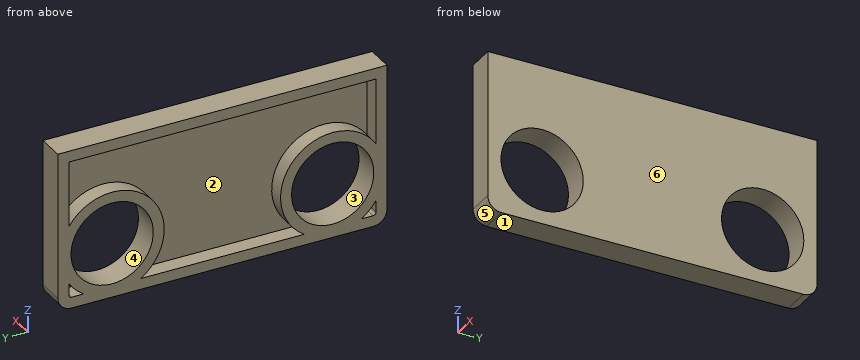
from build123d import *

# Parameters (mm, degrees)
F0_W     = 13.5
F0_H     = 6.75
F1_DEPTH = 20
F2_W     = 8
F2_H     = 26.4694701647
F3_DEPTH = 12
F4_R     = 0.49999
F7_R     = 7.5
F8_DEPTH = 5
F9_T     = -2


# Not quite as in the source:
# - a fillet or chamfer is up to 0.001 mm smaller than in the source, because OpenCascade refuses the exact size
# - a feature of the source that left no trace in its solid (it failed there, or was rolled back) is left out


with BuildPart() as f1:
    # F0 (on Right) → F1 (new body)
    with BuildSketch(Plane.YZ):
        with BuildLine():
            Line((21.2005410668, -21.2570374378), (21.2005410668, 3.4429625622))
            Line((21.2005410668, 3.4429625622), (24.7505410668, 3.4429625622))
            Line((24.7505410668, 3.4429625622), (24.7505410668, -5.3425713437))
            Line((24.7505410668, -5.3425713437), (24.7505410668, -14.0570374378))
            ThreePointArc((24.7505410668, -14.0570374378), (25.4827741138, -15.8248043907), (27.2505410668, -16.5570374378))
            Line((27.2505410668, -16.5570374378), (31.4505410668, -16.5570374378))
            ThreePointArc((31.4505410668, -16.5570374378), (33.2183080197, -15.8248043907), (33.9505410668, -14.0570374378))
            Line((33.9505410668, -14.0570374378), (33.9505410668, -5.3425713437))
            Line((33.9505410668, -5.3425713437), (33.9505410668, 6.3718947504))
            ThreePointArc((33.9505410668, 6.3718947504), (34.4092996144, 7.8152704233), (35.6172077334, 8.7289173543))
            ThreePointArc((35.6172077334, 8.7289173543), (37.4860749727, 16.9784964681), (29.2364958588, 15.1096292289))
            ThreePointArc((29.2364958588, 15.1096292289), (28.3228489279, 13.9017211099), (26.8794732549, 13.4429625622))
            Line((26.8794732549, 13.4429625622), (15.2005410668, 13.4429625622))
            Line((15.2005410668, 13.4429625622), (-1.2994589332, 13.4429625622))
            ThreePointArc((-1.2994589332, 13.4429625622), (-3.0672258862, 12.7107295152), (-3.7994589332, 10.9429625622))
            Line((-3.7994589332, 10.9429625622), (-3.7994589332, 5.9429625622))
            ThreePointArc((-3.7994589332, 5.9429625622), (-3.0672258862, 4.1751956093), (-1.2994589332, 3.4429625622))
            Line((-1.2994589332, 3.4429625622), (5.1650071608, 3.4429625622))
            ThreePointArc((5.1650071608, 3.4429625622), (6.1217157417, 3.2526613935), (6.9327741138, 2.7107295152))
            Line((6.9327741138, 2.7107295152), (14.4934342856, -4.8499306566))
            Line((14.4934342856, -4.8499306566), (15.4683080197, -5.8248043907))
            ThreePointArc((15.4683080197, -5.8248043907), (16.010239898, -6.6358627628), (16.2005410668, -7.5925713437))
            Line((16.2005410668, -7.5925713437), (16.2005410668, -21.2570374378))
            ThreePointArc((16.2005410668, -21.2570374378), (16.4934342856, -21.964144219), (17.2005410668, -22.2570374378))
            Line((17.2005410668, -22.2570374378), (20.2005410668, -22.2570374378))
            ThreePointArc((20.2005410668, -22.2570374378), (20.9076478479, -21.964144219), (21.2005410668, -21.2570374378))
        make_face()
        with Locations((5.7005410668, 7.8179625622)):
            Rectangle(F0_W, F0_H, mode=Mode.SUBTRACT)
    extrude(amount=F1_DEPTH)

    # F2 (on face) → F3 (cut)
    with BuildSketch(Plane.YZ.offset(20)):
        with Locations((5.7005410668, 11.1929625622)):
            Rectangle(F2_W, F2_H)
    extrude(amount=-F3_DEPTH, mode=Mode.SUBTRACT)

    # F4 (radius 0.5 in the source; OpenCascade refuses exactly that, so slightly less here)
    f4_edges = [f1.edges().sort_by_distance(p)[0] for p in [
        (14, 1.700541, 11.192963),
        (14, 1.700541, 13.442963),
        (14, 1.700541, 4.442963),
        (14, 1.700541, 3.442963),
        (10, -1.049459, 4.442963),
        (10, -1.049459, 11.192963),
        (10, 12.450541, 11.192963),
        (10, 12.450541, 4.442963),
        (14, 9.700541, 11.192963),
        (14, 9.700541, 13.442963),
        (14, 9.700541, 4.442963),
    ]]
    fillet(f4_edges, radius=F4_R)


with BuildPart() as f8:
    # F7 (on Right) → F8 (new body)
    with BuildSketch(Plane.YZ):
        with BuildLine():
            Line((-17.6103499532, 45.065652512), (-22.6103499532, 45.065652512))
            Line((-22.6103499532, 45.065652512), (-72.6103499532, 45.065652512))
            Line((-72.6103499532, 45.065652512), (-77.6103499532, 45.065652512))
            Line((-77.6103499532, 45.065652512), (-77.6103499532, 27.565652512))
            ThreePointArc((-77.6103499532, 27.565652512), (-76.8781169061, 25.7978855591), (-75.1103499532, 25.065652512))
            Line((-75.1103499532, 25.065652512), (-20.1103499532, 25.065652512))
            ThreePointArc((-20.1103499532, 25.065652512), (-18.3425830002, 25.7978855591), (-17.6103499532, 27.565652512))
            Line((-17.6103499532, 27.565652512), (-17.6103499532, 45.065652512))
        make_face()
        with Locations((-67.7103499532, 35.015652512)):
            Circle(F7_R, mode=Mode.SUBTRACT)
        with Locations((-27.5103499532, 35.015652512)):
            Circle(F7_R, mode=Mode.SUBTRACT)
        Polygon((-72.6103499532, 45.065652512), (-22.6103499532, 45.065652512), (-17.6103499532, 45.065652512), (-17.6103499532, 54.265652512), (-77.6103499532, 54.265652512), (-77.6103499532, 45.065652512), align=None)
    extrude(amount=F8_DEPTH)

    # F9
    f9_openings = [f8.faces().sort_by_distance(p)[0] for p in [
        (0, -47.61035, 40.869984),
    ]]
    offset(amount=F9_T, openings=f9_openings)


solid = f8.part
Read the model definition and answer for the solid it produces. Units are mm, in the model's axes. Face numbers are marked on the shaded views. A direction names the side the tool comes from. Round coordinates to 2 decimals unless told otherwise and drop trailing zeros. Order: outer loops, then holes, each group sorted by start corner. A loop starts at its lowest first (then second) coordinate and runs counter-clockwise, first axis right, second up.
1) Flat-ended cylindrical pins translate along their axes: pin 1 (7.5 mm diameter, centred on y = -55.5, z = 41.5, fed in from -X); pin 2 (9 mm diameter, centred on y = -27.51, z = 35.02, fed in from -X). Find the tip coordinate at first contact, or state that the pin passes through.
2) Straight lines are drawn through the part: L1, parallel to Z at x = 2.1, y = -68; L2, parallel to Z at x = 0.3, y = -34; L3, parallel to Z at x = 1.5, y = -62. For each, find the intervals that lie inside material, in ascending order.
3) For the marked faces 1 and 2, determine the directions among +Z, -Z, +X, -X, +Y, -Y from which every point of the face is accessible in a straight line to the end or side of a thin tool.
4) The part is cut by section A-A on z = 33. Write down the section's boundary in (x, y), plus the area to 3 significant figures.
5) The part is cut by section D-D on y = -49.5. Write down the section's boundary in (x, z).
6) The part is cut by section B-B on y = -74. Write down the section's boundary in (x, z), plus the area to 3 significant figures.
7) The mould has two halves that part along Y. Classify the marked faces 3, 4, 5 and 6: released by +Y, released by -Y, zero draft, split by the parting line, or undercut.
8) The part is cut by section C-C on x = 0.6. Write down the section's boundary in (y, z), plus the area to 3 significant figures.
Resolved:
1. pin 1: stops at x = 3
1. pin 2: passes through
2. L1: z = 25.07 to 27.52, 42.51 to 44.51, 52.27 to 54.27
2. L2: z = 25.07 to 27.07, 28.08 to 31.26, 38.78 to 41.95, 52.27 to 54.27
2. L3: z = 25.07 to 27.07, 27.42 to 30.15, 39.88 to 42.61, 52.27 to 54.27
3. face 1: -Z, +X, -X, +Y, -Y
3. face 2: -X
4. outline: (0, -77.61) - (5, -77.61) - (5, -74.93) - (0, -74.93) - close; (0, -60.49) - (5, -60.49) - (5, -34.73) - (0, -34.73) - (0, -36.79) - (3, -36.79) - (3, -58.43) - (0, -58.43) - close; (0, -20.29) - (5, -20.29) - (5, -17.61) - (0, -17.61) - close
4. area: 90.6 mm2
5. outline: (0, 25.07) - (5, 25.07) - (5, 54.27) - (0, 54.27) - (0, 52.27) - (3, 52.27) - (3, 27.07) - (0, 27.07) - close
6. outline: (0, 25.07) - (5, 25.07) - (5, 30.93) - (0, 30.93) - (0, 27.9) - (3, 27.9) - (3, 27.07) - (0, 27.07) - close; (0, 39.1) - (5, 39.1) - (5, 54.27) - (0, 54.27) - (0, 52.27) - (3, 52.27) - (3, 42.14) - (0, 42.14) - close
6. area: 72.3 mm2
7. face 3: undercut
7. face 4: undercut
7. face 5: released by -Y
7. face 6: zero draft
8. outline: (-77.61, 27.57) arc R2.5 ccw to (-75.11, 25.07) - (-20.11, 25.07) arc R2.5 ccw to (-17.61, 27.57) - (-17.61, 54.27) - (-77.61, 54.27) - close; hole (-75.61, 27.57) arc R0.5 ccw to (-75.11, 27.07) - (-72.91, 27.07) arc R9.5 cw to (-75.61, 29.74) - close; hole (-75.61, 40.29) arc R9.5 cw (long way) to (-62.51, 27.07) - (-32.71, 27.07) arc R9.5 cw (long way) to (-19.61, 40.29) - (-19.61, 52.27) - (-75.61, 52.27) - close; hole circle Ø15 at (-67.71, 35.02); hole circle Ø15 at (-27.51, 35.02); hole (-22.31, 27.07) - (-20.11, 27.07) arc R0.5 ccw to (-19.61, 27.57) - (-19.61, 29.74) arc R9.5 cw to start
8. area: 507 mm2
